```python
from build123d import *

# Parameters (mm, degrees)
SKETCH004_W     = 66.78
SKETCH004_H     = 112
PAD002_DEPTH    = 4
SKETCH005_W     = 62.78
SKETCH005_H     = 108
PAD003_DEPTH    = 15.3
SKETCH006_W     = 62.78
SKETCH006_H     = 108
POCKET002_DEPTH = 2
SKETCH007_W     = 58.78
SKETCH007_H     = 104
POCKET003_DEPTH = 15.3
SKETCH008_R     = 3.5
PAD004_DEPTH    = 14.5
SKETCH009_R     = 2.5
PAD005_DEPTH    = 0.8
SKETCH010_W     = 31.5
SKETCH010_H     = 5.15
POCKET004_DEPTH = 5
SKETCH011_W     = 31
SKETCH011_H     = 15
POCKET005_DEPTH = 5


with BuildPart() as part:
    # Sketch004 → Pad002 (new body)
    with BuildSketch(Plane.XY):
        with Locations((31.39, 54)):
            Rectangle(SKETCH004_W, SKETCH004_H)
    extrude(amount=-PAD002_DEPTH)

    # Sketch005 (on Face5 of Pad002) → Pad003 (join)
    with BuildSketch(Plane.XY):
        with Locations((31.39, 54)):
            Rectangle(SKETCH005_W, SKETCH005_H)
    extrude(amount=PAD003_DEPTH)

    # Sketch006 (on Face5 of Pad003) → Pocket002 (cut)
    with BuildSketch(Plane(origin=(0, 0, -4), x_dir=(1, 0, 0), z_dir=(0, 0, -1))):
        with Locations((31.39, -54)):
            Rectangle(SKETCH006_W, SKETCH006_H)
    extrude(amount=-POCKET002_DEPTH, mode=Mode.SUBTRACT)

    # Sketch007 (on Face16 of Pocket002) → Pocket003 (cut)
    with BuildSketch(Plane(origin=(0, 0, -2), x_dir=(1, 0, 0), z_dir=(0, 0, -1))):
        with Locations((31.39, -54)):
            Rectangle(SKETCH007_W, SKETCH007_H)
    extrude(amount=-POCKET003_DEPTH, mode=Mode.SUBTRACT)

    # Sketch008 (on Face21 of Pocket003) → Pad004 (join)
    with BuildSketch(Plane(origin=(0, 0, 13.3), x_dir=(1, 0, 0), z_dir=(0, 0, -1))):
        with Locations((7, -7)):
            Circle(SKETCH008_R)
        with Locations((47, -7)):
            Circle(SKETCH008_R)
        with Locations((7, -101)):
            Circle(SKETCH008_R)
        with Locations((47, -101)):
            Circle(SKETCH008_R)
    extrude(amount=PAD004_DEPTH)

    # Sketch009 (on Face28 of Pad004) → Pad005 (join)
    with BuildSketch(Plane(origin=(0, 0, -1.2), x_dir=(1, 0, 0), z_dir=(0, 0, -1))):
        with Locations((7, -7)):
            Circle(SKETCH009_R)
        with Locations((47, -7)):
            Circle(SKETCH009_R)
        with Locations((7, -101)):
            Circle(SKETCH009_R)
        with Locations((47, -101)):
            Circle(SKETCH009_R)
    extrude(amount=PAD005_DEPTH)

    # Sketch010 (on Face3 of Pad005) → Pocket004 (cut)
    with BuildSketch(Plane.YZ.offset(64.78)):
        with Locations((74.75, -4.575)):
            Rectangle(SKETCH010_W, SKETCH010_H)
    extrude(amount=-POCKET004_DEPTH, mode=Mode.SUBTRACT)

    # Sketch011 (on Face3 of Pocket004) → Pocket005 (cut)
    with BuildSketch(Plane.YZ.offset(64.78)):
        with Locations((26, 3.5)):
            Rectangle(SKETCH011_W, SKETCH011_H)
    extrude(amount=-POCKET005_DEPTH, mode=Mode.SUBTRACT)


solid = part.part
```
Check sheet for the modelled part. Datum: model origin and axes. Units: mm. A direction names the side the tool comes from. Round coordinates to 2 decimals unless told otherwise and drop trailing zeros. Write each loop counter-clockwise with the first axis right and the second up, starting at its lowest first coordinate (ties: lowest second). Pieces come first, ordered by that corner, then holes. Notation, with made-up numbers: (69.25, 17) -> (74.25, 17) arc R17 cw to (74.25, 49) -> close; hole circle Ø2 at (-21.5, -28). An arc over 180 degrees is marked (long way). One line per question, with ' | ' between items. Start each with the question number.
1. Sectioned sample at A-A, the plane z = 2.5. Record the cut outline in (x, y), then the cut area to 3 significant figures.
2. Sectioned sample at C-C, the plane y = 60.5. Record the cut outline in (x, z), then the cut area to 3 significant figures.
3. Depth check by flat-ended pin: pin 1 (3 mm diameter, centred on y = 33.5, z = 10, fed in from -X); pin 2 (4 mm diameter, centred on x = 46.5, y = 100.5, fed in from -Z); pin 3 (1.2 mm diameter, centred on x = 62.5, z = 6.5, fed in from +Y). Enter the tip coordinate at first touch or a pass-through.
4. Scan lines: line 1 along X through (y, z) = (89.5, 8.5); line 2 along Y through (x, z) = (58, 8.5); line 3 along X through (y, z) = (6.5, 6). Record each from-to range of solid material in increasing order. Write a range as from..to.
5. Sectioned sample at B-B, the plane x = 19. Record the cut outline in (y, z), then the cut area to 3 significant figures.
6. Release check for a two-part mould opening along X. For faces 1 (the face through (31, 106, 6)), 2 (the face through (-1, 79, -4)), 3 (the face through (64.78, 4, -2)) record: +X half, -X half, draft (parallel to the pull), parting line (faces both ways), or undercut.
7. Set-up check for faces 4 (the face through (31, -2, -2)), 5 (the face through (9, 9, -1.2)): record each of +Z, -Z, +X, -X, +Y, -Y from which the full face is reachable in a straight line by a thin tool's end or side.
Taken from the geometry:
1) outline: (0, 0) -> (62.78, 0) -> (62.78, 10.5) -> (60.78, 10.5) -> (60.78, 2) -> (2, 2) -> (2, 106) -> (60.78, 106) -> (60.78, 41.5) -> (62.78, 41.5) -> (62.78, 108) -> (0, 108) -> close; circle Ø7 at (7, 7); circle Ø7 at (7, 101); circle Ø7 at (47, 7); circle Ø7 at (47, 101) | area: 759 mm^2
2) outline: (-2, -4) -> (0, -4) -> (0, -2) -> (2, -2) -> (2, 13.3) -> (60.78, 13.3) -> (60.78, -2) -> (64.78, -2) -> (64.78, 0) -> (62.78, 0) -> (62.78, 15.3) -> (0, 15.3) -> (0, 0) -> (-2, 0) -> close | area: 199 mm^2
3) pin 1: stops at x = 0 | pin 2: stops at z = -2 | pin 3: stops at y = 108
4) line 1: x = 0..2, 60.78..62.78 | line 2: y = 0..2, 106..108 | line 3: x = 0..2, 3.54..10.46, 43.54..50.46, 60.78..62.78
5) outline: (-2, -4) -> (0, -4) -> (0, -2) -> (2, -2) -> (2, 13.3) -> (106, 13.3) -> (106, -2) -> (108, -2) -> (108, -4) -> (110, -4) -> (110, 0) -> (108, 0) -> (108, 15.3) -> (0, 15.3) -> (0, 0) -> (-2, 0) -> close | area: 293 mm^2
6) face 1: undercut | face 2: draft | face 3: +X half
7) face 4: +Z, -Z, +X, -X, -Y | face 5: -Z
